```python
from build123d import *

# Parameters (mm, degrees)
SKETCH1_R           = 9.525
BOSS_EXTRUDE1_DEPTH = 508
DOME1_FACE_RADIUS   = 9.525
DOME1_HEIGHT        = 6.35


# Read off the part's stored shape, not the designer's step: Shell1
with BuildPart() as part:
    # Sketch1 → Boss-Extrude1 (new body)
    with BuildSketch(Plane(origin=(0, 0, 0), x_dir=(0, 0, -1), z_dir=(1, 0, 0))):
        Circle(SKETCH1_R)
    extrude(amount=-BOSS_EXTRUDE1_DEPTH)

    # Dome1: a dome of height H over a round flat face of radius A is a cap of a sphere of radius (A * A + H * H) / (2 * H)
    dome1_r = (DOME1_FACE_RADIUS * DOME1_FACE_RADIUS + DOME1_HEIGHT * DOME1_HEIGHT) / (2 * DOME1_HEIGHT)
    dome1_base = Plane((-508, 0, 0), z_dir=(-1, 0, 0))
    with Locations(dome1_base.offset(DOME1_HEIGHT - dome1_r)):
        dome1_ball = Sphere(dome1_r, mode=Mode.PRIVATE)
    add(split(dome1_ball, bisect_by=dome1_base, keep=Keep.TOP, mode=Mode.PRIVATE))

    # Shell1 outline → Shell1 (revolve, cut)
    with BuildSketch(Plane.YX):
        with BuildLine():
            ThreePointArc((0, -511.81), (4.115838187, -510.631918722), (6.985000003, -507.454512554))
            Line((6.985000003, -507.454512554), (6.985, 0))
            Line((6.985, 0), (0, 0))
            Line((0, 0), (0, -511.81))
        make_face()
    revolve(axis=Axis((0, 0, 0), (1, 0, 0)), mode=Mode.SUBTRACT)


solid = part.part
```
Verification items for the finished model (mm, model axes). Give positions to 0.01 mm unless a question says otherwise; leave off trailing zeros. Order: outer loops, then holes, each group sorted by start corner. A loop starts at its lowest first (then second) coordinate and runs counter-clockwise, first axis right, second up. Notation, with made-up numbers: (70, 65.5) -> (106, 65.5) arc R23 cw to (106, 103.5) -> close; hole circle Ø2 at (84.5, 85). An arc over 180 degrees is marked (long way). One line per item, written item: value.
(1) Sectioned sample at C-C on x = -100.5. Record the cut outline in (y, z) (3 decimals).
Final values:
outline: circle Ø19.05 at (0, 0); hole circle Ø13.97 at (0, 0)
(2) Scan lines: line 1 along Z through (x, y) = (-145, -1); line 2 along Y through (x, z) = (-413, -0.25); line 3 along Z through (x, y) = (-229, 3.25). Record each from-to range of solid material in increasing order. Write a range as [from, to].
Final values:
line 1: [-9.47, -6.91], [6.91, 9.47]
line 2: [-9.52, -6.98], [6.98, 9.52]
line 3: [-8.95, -6.18], [6.18, 8.95]
(3) Gauge pin test, flat ends, axial feed: pin 1 (1.5 mm diameter, centred on x = -398, y = 1, fed in from -Z); pin 2 (4 mm diameter, centred on x = -442.5, y = 6, fed in from -Z); pin 3 (4 mm diameter, centred on x = -337.5, z = -6.5, fed in from +Y) (3 decimals). Record the tip position at first contact, or that the pin passes through.
Final values:
pin 1: z = -9.52
pin 2: z = -8.64
pin 3: y = 8.395
(4) Draft check along Z on faces 1 (the face through (-250.444, -5.796, 7.559)), 2 (the face through (-250.175, -0.909, 6.926)), 3 (the face through (0, 7.1, 0.8)). Enter one of: pulls with the +Z half, pulls with the -Z half, needs draft (parallel to the pull), parting line crosses it, or undercut.
Final values:
face 1: parting line crosses it
face 2: undercut
face 3: needs draft
(5) Sectioned sample at A-A on z = 0. Record the cut outline in (x, y) (1 decimal).
Final values:
outline: (-508, -9.5) -> (0, -9.5) -> (0, -7) -> (-507.5, -7) arc R7.8 cw to (-507.5, 7) -> (0, 7) -> (0, 9.5) -> (-508, 9.5) arc R10.3 ccw to start
